Check sheet for the modelled part. Datum: model origin and axes. Units: mm. A direction names the side the tool comes from. Coordinates: 2 decimals unless noted, no trailing zeros. Loops run counter-clockwise (first coordinate to the right, second up) from the corner with the lowest first, then second, coordinate; pieces in that order, holes last. Notation, with made-up numbers: (-19, 76.5) - (16, 76.5) arc R25 ccw to (16, 93.5) - close; hole circle Ø3 at (-22, 20.5). An arc over 180 degrees is marked (long way). Write each question's results on one line, items separated by ' | '. Start each with the question number.
1. Thickness scan on line 1 (X direction, y = 1.2, z = 13); line 2 (Z direction, x = -6, y = 0.75); line 3 (Z direction, x = 3, y = 1.35). Record the ranges inside material, lowest first. Write a range as [from, to].
2. Cross-section at B-B (y = 1.1). Record the cut outline in (x, z).
3. Tool access check on faces 5 (the face through (-2.953, 1.479, 5.434)), 6 (the face through (-9, 1, 5)). Record the directions out of +Z, -Z, +X, -X, +Y, -Y that give a thin tool (end or side, any length) a straight path to the whole face; none if there is none.
4. Cross-section at D-D (z = -2.75). Record the cut outline in (x, y).
5. Draft check along Z on faces 1 (the face through (-5.845, 1.479, -0.803)), 2 (the face through (0, 1, 15.5)), 3 (the face through (0, 0, 10)), 4 (the face through (-6, 1, -5.4)). Enter one of: released by +Z, released by -Z, zero draft, split by the parting line, or undercut.
6. Cross-section at A-A (z = 13). Record the cut outline in (x, y).
7. Cross-section at C-C (x = -3). Record the cut outline in (y, z).
```python
from build123d import *

# Parameters (mm, degrees)
CROQUIS1_R              = 1.4
SALIENTE_EXTRUIR1_DEPTH = 3


with BuildPart() as part:
    # Croquis1 → Saliente-Extruir1 (new body)
    with BuildSketch(Plane(origin=(0, 0, 0), x_dir=(1, 0, 0), z_dir=(0, 1, 0))):
        with BuildLine():
            Line((2.376972865, 5.4), (9, 5.4))
            Line((9, 5.4), (9, -15.5))
            Line((9, -15.5), (-9, -15.5))
            Line((-9, -15.5), (-9, 5.4))
            Line((-9, 5.4), (-2.376972865, 5.4))
            ThreePointArc((-2.376972865, 5.4), (-5.856174249, 0.717790472), (-3.610771276, -4.666083025))
            ThreePointArc((-3.610771276, -4.666083025), (-2.945738566, -5.446622945), (-2.65, -6.428483309))
            ThreePointArc((-2.65, -6.428483309), (0, -8.859831691), (2.65, -6.428483309))
            ThreePointArc((2.65, -6.428483309), (2.945738566, -5.446622945), (3.610771276, -4.666083025))
            ThreePointArc((3.610771276, -4.666083025), (5.856174249, 0.717790472), (2.376972865, 5.4))
        make_face()
        with Locations((-6, -13)):
            Circle(CROQUIS1_R, mode=Mode.SUBTRACT)
        with Locations((6, -13)):
            Circle(CROQUIS1_R, mode=Mode.SUBTRACT)
    extrude(amount=SALIENTE_EXTRUIR1_DEPTH)


solid = part.part
```
Established:
1) line 1: [-9, -7.4], [-4.6, 4.6], [7.4, 9] | line 2: [-5.4, 11.6], [14.4, 15.5] | line 3: [-5.4, -5.08], [5.35, 15.5]
2) outline: (-9, -5.4) - (-2.38, -5.4) arc R5.9 cw to (-3.61, 4.67) arc R2.5 ccw to (-2.65, 6.43) arc R2.66 cw to (2.65, 6.43) arc R2.5 ccw to (3.61, 4.67) arc R5.9 cw to (2.38, -5.4) - (9, -5.4) - (9, 15.5) - (-9, 15.5) - close; hole circle Ø2.8 at (-6, 13); hole circle Ø2.8 at (6, 13)
3) face 5: +Y, -Y | face 6: +Z, -Z, -X, +Y, -Y
4) outline: (-9, 0) - (-5.22, 0) - (-5.22, 3) - (-9, 3) - close; (5.22, 0) - (9, 0) - (9, 3) - (5.22, 3) - close
5) face 1: undercut | face 2: released by +Z | face 3: zero draft | face 4: released by -Z
6) outline: (-9, 0) - (-7.4, 0) - (-7.4, 3) - (-9, 3) - close; (-4.6, 0) - (4.6, 0) - (4.6, 3) - (-4.6, 3) - close; (7.4, 0) - (9, 0) - (9, 3) - (7.4, 3) - close
7) outline: (0, -5.4) - (3, -5.4) - (3, -5.08) - (0, -5.08) - close; (0, 5.35) - (3, 5.35) - (3, 15.5) - (0, 15.5) - close
